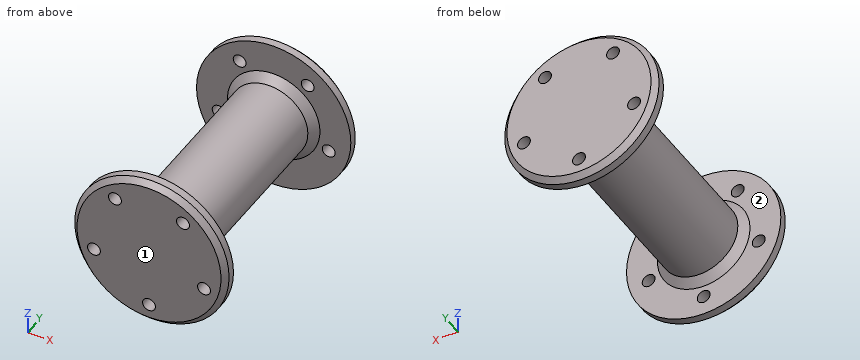
```python
from build123d import *

# Parameters (mm, degrees)
SKETCH1_R                = 15
BOSS_EXTRUDE1_DEPTH      = 40
SKETCH4_R                = 30
BOSS_EXTRUDE2_DEPTH      = 5
CHAMFER1_SIZE            = 2
SKETCH6_R                = 2.5
CUT_EXTRUDE1_DEPTH       = 96
CIRPATTERN1_COUNT        = 5
CHAMFER2_SIZE            = 3
MIRROR1_COPY_1_SKETCH_R  = 2.5
MIRROR1_COPY_1_DEPTH     = 96
MIRROR1_COPY_2_SKETCH_R  = 2.5
MIRROR1_COPY_2_DEPTH     = 96
MIRROR1_COPY_3_SKETCH_R  = 2.5
MIRROR1_COPY_3_DEPTH     = 96
MIRROR1_COPY_4_SKETCH_R  = 2.5
MIRROR1_COPY_4_DEPTH     = 96
MIRROR1_COPY_5_SKETCH_R  = 2.5
MIRROR1_COPY_5_DEPTH     = 96
CHAMFER1_OF_MIRROR1_SIZE = 2
CHAMFER2_OF_MIRROR1_SIZE = 3


with BuildPart() as part:
    # Sketch1 → Boss-Extrude1 (new, symmetric)
    with BuildSketch(Plane(origin=(0, 0, 0), x_dir=(1, 0, 0), z_dir=(0, 1, 0))):
        with Locations(Location((0, 0, 0), (0, 0, 270))):
            Circle(SKETCH1_R)
    extrude(amount=BOSS_EXTRUDE1_DEPTH, both=True)

    # Sketch4 → Boss-Extrude2 (add)
    with BuildSketch(Plane(origin=(0, 40, 0), x_dir=(1, 0, 0), z_dir=(0, 1, 0))):
        with Locations(Location((0, 0, 0), (0, 0, 270))):
            Circle(SKETCH4_R)
    boss_extrude2 = extrude(amount=BOSS_EXTRUDE2_DEPTH)

    # Chamfer1
    chamfer1_edges = [part.edges().sort_by_distance(p)[0] for p in [
        (0, 45, -30),
    ]]
    chamfer(chamfer1_edges, length=CHAMFER1_SIZE)

    # Sketch6 → Cut-Extrude1 (cut, through all)
    with BuildSketch(Plane(origin=(0, 45, 0), x_dir=(1, 0, 0), z_dir=(0, 1, 0))):
        with Locations(Location((0, 22.5, 0), (0, 0, 270))):
            Circle(SKETCH6_R)
    cut_extrude1 = extrude(amount=-CUT_EXTRUDE1_DEPTH, mode=Mode.SUBTRACT)

    # CirPattern1: Cut-Extrude1 ×5 about axis
    cirpattern1_axis = Axis((0, 0, 0), (0, 1, 0))
    for i in range(1, CIRPATTERN1_COUNT):
        add(cut_extrude1.rotate(cirpattern1_axis, i * 360 / CIRPATTERN1_COUNT), mode=Mode.SUBTRACT)

    # Chamfer2
    chamfer2_edges = [part.edges().sort_by_distance(p)[0] for p in [
        (0, 40, -15),
    ]]
    chamfer(chamfer2_edges, length=CHAMFER2_SIZE)

    # Mirror1: Boss-Extrude2 across plane
    add(boss_extrude2.mirror(Plane.ZX))

    # Mirror1 copy 1 sketch → Mirror1 copy 1 (cut, through all)
    with BuildSketch(Plane(origin=(0, -45, 0), x_dir=(0.30901699437494745, 0, -0.9510565162951535), z_dir=(0, -1, 0))):
        with Locations((0, -22.5)):
            Circle(MIRROR1_COPY_1_SKETCH_R)
    extrude(amount=-MIRROR1_COPY_1_DEPTH, mode=Mode.SUBTRACT)

    # Mirror1 copy 2 sketch → Mirror1 copy 2 (cut, through all)
    with BuildSketch(Plane(origin=(0, -45, 0), x_dir=(-0.8090169943749473, 0, -0.5877852522924732), z_dir=(0, -1, 0))):
        with Locations((0, -22.5)):
            Circle(MIRROR1_COPY_2_SKETCH_R)
    extrude(amount=-MIRROR1_COPY_2_DEPTH, mode=Mode.SUBTRACT)

    # Mirror1 copy 3 sketch → Mirror1 copy 3 (cut, through all)
    with BuildSketch(Plane(origin=(0, -45, 0), x_dir=(-0.8090169943749476, 0, 0.587785252292473), z_dir=(0, -1, 0))):
        with Locations((0, -22.5)):
            Circle(MIRROR1_COPY_3_SKETCH_R)
    extrude(amount=-MIRROR1_COPY_3_DEPTH, mode=Mode.SUBTRACT)

    # Mirror1 copy 4 sketch → Mirror1 copy 4 (cut, through all)
    with BuildSketch(Plane(origin=(0, -45, 0), x_dir=(0.30901699437494723, 0, 0.9510565162951536), z_dir=(0, -1, 0))):
        with Locations((0, -22.5)):
            Circle(MIRROR1_COPY_4_SKETCH_R)
    extrude(amount=-MIRROR1_COPY_4_DEPTH, mode=Mode.SUBTRACT)

    # Mirror1 copy 5 sketch → Mirror1 copy 5 (cut, through all)
    with BuildSketch(Plane.XZ.offset(45)):
        with Locations((0, -22.5)):
            Circle(MIRROR1_COPY_5_SKETCH_R)
    extrude(amount=-MIRROR1_COPY_5_DEPTH, mode=Mode.SUBTRACT)

    # Chamfer1 of Mirror1
    chamfer1_of_mirror1_edges = [part.edges().sort_by_distance(p)[0] for p in [
        (0, -45, -30),
    ]]
    chamfer(chamfer1_of_mirror1_edges, length=CHAMFER1_OF_MIRROR1_SIZE)

    # Chamfer2 of Mirror1
    chamfer2_of_mirror1_edges = [part.edges().sort_by_distance(p)[0] for p in [
        (0, -40, -15),
    ]]
    chamfer(chamfer2_of_mirror1_edges, length=CHAMFER2_OF_MIRROR1_SIZE)


solid = part.part
```
The listing builds one solid part. Answer for the finished solid, in the listing's coordinates (mm). Face numbers are marked on the shaded views. A direction names the side the tool comes from. Give positions to 0.01 mm unless a question says otherwise; leave off trailing zeros. Order: outer loops, then holes, each group sorted by start corner. A loop starts at its lowest first (then second) coordinate and runs counter-clockwise, first axis right, second up. Notation, with made-up numbers: (48, 64.5) - (98, 64.5) arc R29 cw to (98, 88.5) - close; hole circle Ø1 at (-5, 29). An arc over 180 degrees is marked (long way). Answer in a Markdown table with one row per item. Add a question column.
Q1. Given P1, Ø5, axis at y = 13.5, z = -9, coming from the +X side; P2, Ø8, axis at y = -21.5, z = 17, coming from the +X side; P3, Ø1.5, axis at y = 28, z = -0.5, coming from the +X side, each flat-ended and moving along its own axis, determine where each tip first touches the part or whether it passes through.
Q2. The part is cut by section B-B (z = 0). Determine the outline of the cut face in (x, y).
Q3. The part is cut by section D-D (y = -7). Determine the outline of the cut face in (x, z).
Q4. The part is cut by section C-C (z = -22.5). Give the number of separate pieces and of enclosed holes in the cut face, then the cut area to 3 significant figures.
Q5. The part is cut by section A-A (x = 0). Determine the outline of the cut face in (y, z), then the cut area to 3 significant figures.
Q6. Find the intervals of material crossed by line 1 along Y through (x, z) = (3, -25); line 2 along X through (y, z) = (-40.5, 16.5); line 3 along Y through (x, z) = (-9, 15.5), in increasing order. Write a range as [from, to].
Q7. Which of the six approach directions +Z, -Z, +X, -X, +Y, -Y give full straight-line access (tool end or side, diameter ignored) to the marked faces 1 and 2?
Determined:
| question | item | result |
|---|---|---|
| 1 | P1 | stops at x = 13.52 |
| 1 | P2 | stops at x = 7.48 |
| 1 | P3 | stops at x = 15 |
| 2 | outline | (-30, -43) - (-28, -45) - (28, -45) - (30, -43) - (30, -40) - (18, -40) - (15, -37) - (15, 37) - (18, 40) - (30, 40) - (30, 43) - (28, 45) - (-28, 45) - (-30, 43) - (-30, 40) - (-18, 40) - (-15, 37) - (-15, -37) - (-18, -40) - (-30, -40) - close |
| 3 | outline | circle Ø30 at (0, 0) |
| 4 | separate pieces | 4 |
| 4 | enclosed holes | 0 |
| 4 | area | 334 mm² |
| 5 | outline | (-45, -28) - (-43, -30) - (-40, -30) - (-40, -25) - (-45, -25) - close; (-45, -20) - (-40, -20) - (-40, -18) - (-37, -15) - (37, -15) - (40, -18) - (40, -20) - (45, -20) - (45, 28) - (43, 30) - (40, 30) - (40, 18) - (37, 15) - (-37, 15) - (-40, 18) - (-40, 30) - (-43, 30) - (-45, 28) - close; (40, -30) - (43, -30) - (45, -28) - (45, -25) - (40, -25) - close |
| 5 | area | 2,960 mm² |
| 6 | line 1 | y = [-45, -40], [40, 45] |
| 6 | line 2 | x = [-25.05, -15.06], [-11.39, 11.39], [15.06, 25.05] |
| 6 | line 3 | y = [-45, -39.92], [39.92, 45] |
| 7 | face 1 | +Z, -Z, +X, -X, -Y |
| 7 | face 2 | none |
